Check sheet for the modelled part. Datum: model origin and axes. Units: mm. A direction names the side the tool comes from. Give positions to 0.01 mm unless a question says otherwise; leave off trailing zeros. Order: outer loops, then holes, each group sorted by start corner. A loop starts at its lowest first (then second) coordinate and runs counter-clockwise, first axis right, second up. Notation, with made-up numbers: (31, -9.75) -> (77, -9.75) arc R17 cw to (77, -5.75) -> close; hole circle Ø11 at (16, 29.25). An arc over 180 degrees is marked (long way). One line per question, with ' | ' between items.
```python
from build123d import *

# Parameters (mm, degrees)
AUFSATZ_LINEAR_AUSTRAGEN3_DEPTH      = 20
SKIZZE10_OUTSIDE_W                   = 46.486
SKIZZE10_OUTSIDE_H                   = 31.486
SCHNITT_LINEAR_AUSTRAGEN9_DEPTH      = 13.5
SCHNITT_LINEAR_AUSTRAGEN9_DEPTH_BACK = 13.5
SKIZZE7_R                            = 1.23
SCHNITT_LINEAR_AUSTRAGEN8_DEPTH      = 12


with BuildPart() as part:
    # Skizze3 → Aufsatz-Linear austragen3 (new body)
    with BuildSketch(Plane.XY):
        with BuildLine():
            Line((-17.5, 4), (-2.308809744, 11.933429348))
            ThreePointArc((-2.308809744, 11.933429348), (0, 12.5), (2.308809744, 11.933429348))
            Line((2.308809744, 11.933429348), (17.5, 4))
            Line((17.5, 4), (17.5, -4))
            Line((17.5, -4), (2.308809744, -11.933429348))
            ThreePointArc((2.308809744, -11.933429348), (0, -12.5), (-2.308809744, -11.933429348))
            Line((-2.308809744, -11.933429348), (-17.5, -4))
            Line((-17.5, -4), (-17.5, 4))
        make_face()
        with BuildLine():
            Line((-2.25, -7.51244486), (-2.25, 7.51244486))
            ThreePointArc((-2.25, 7.51244486), (0, 9.76244486), (2.25, 7.51244486))
            Line((2.25, 7.51244486), (2.25, -7.51244486))
            ThreePointArc((2.25, -7.51244486), (0, -9.76244486), (-2.25, -7.51244486))
        make_face(mode=Mode.SUBTRACT)
    extrude(amount=AUFSATZ_LINEAR_AUSTRAGEN3_DEPTH)

    # Skizze10 outside → Schnitt-Linear austragen9 (cut, two sides)
    with BuildSketch(Plane(origin=(0, 0, 0), x_dir=(1, 0, 0), z_dir=(0, 1, 0))) as schnitt_linear_austragen9_sk:
        with Locations((0, -10)):
            Rectangle(SKIZZE10_OUTSIDE_W, SKIZZE10_OUTSIDE_H)
        with BuildLine():
            Line((-16.110814579, 0), (-17.5, -7.878462024))
            Line((-17.5, -7.878462024), (-3.472963553, -10.351807009))
            ThreePointArc((-3.472963553, -10.351807009), (0, -10.655651949), (3.472963553, -10.351807009))
            Line((3.472963553, -10.351807009), (17.5, -7.878462024))
            Line((17.5, -7.878462024), (16.110814579, 0))
            Line((16.110814579, 0), (-16.110814579, 0))
        make_face(mode=Mode.SUBTRACT)
    extrude(amount=SCHNITT_LINEAR_AUSTRAGEN9_DEPTH, mode=Mode.SUBTRACT)
    extrude(schnitt_linear_austragen9_sk.sketch, amount=-SCHNITT_LINEAR_AUSTRAGEN9_DEPTH_BACK, mode=Mode.SUBTRACT)

    # Skizze7 → Schnitt-Linear austragen8 (cut)
    with BuildSketch(Plane(origin=(-16.983254832, 0, 4.947854546), x_dir=(-0.173648178, 0, 0.984807753), z_dir=(-0.984807753, 0, -0.173648178))):
        with Locations((-1.524183177, 0)):
            Circle(SKIZZE7_R)
    schnitt_linear_austragen8 = extrude(amount=-SCHNITT_LINEAR_AUSTRAGEN8_DEPTH, mode=Mode.SUBTRACT)

    # Spiegeln4: Schnitt-Linear austragen8 across plane
    add(schnitt_linear_austragen8.mirror(Plane(origin=(0, 0, 0), x_dir=(0, 0, 1), z_dir=(1, 0, 0))), mode=Mode.SUBTRACT)


solid = part.part
```
Q1. Section check B-B (y = 2.5). Enter the section's corners in (x, z), and give its area (3 significant figures).
Result sheet:
outline: (-17.5, 7.88) -> (-16.11, 0) -> (-2.25, 0) -> (-2.25, 10.53) arc R20 ccw to (-3.47, 10.35) -> close; (2.25, 0) -> (16.11, 0) -> (17.5, 7.88) -> (3.47, 10.35) arc R20 ccw to (2.25, 10.53) -> close | area: 270 mm2
Q2. Depth check by flat-ended pin: pin 1 Ø1 at (y, z) = (8, 5.5) entering from +X; pin 2 Ø6 at (x, z) = (1, 5) entering from +Y; pin 3 Ø5 at (x, z) = (6.5, 5.5) entering from +Y; pin 4 Ø3 at (y, z) = (1, 4) entering from +X. Enter the tip coordinate at first touch or a pass-through.
Result sheet:
pin 1: stops at x = 10.8 | pin 2: stops at y = 12.5 | pin 3: stops at y = 11.05 | pin 4: stops at x = 17.08
Q3. Section check A-A (x = 0). Enter the section's corners in (y, z), and give its area (3 significant figures).
Result sheet:
outline: (-12.5, 0) -> (-9.76, 0) -> (-9.76, 10.66) -> (-12.5, 10.66) -> close; (9.76, 0) -> (12.5, 0) -> (12.5, 10.66) -> (9.76, 10.66) -> close | area: 58.3 mm2
Q4. Section check C-C (z = 9.75). Enter the section's corners in (x, y), and give its area (3 significant figures).
Result sheet:
outline: (-6.89, -9.54) -> (-2.31, -11.93) arc R4.99 ccw to (2.31, -11.93) -> (6.89, -9.54) -> (6.89, 9.54) -> (2.31, 11.93) arc R4.99 ccw to (-2.31, 11.93) -> (-6.89, 9.54) -> close; hole (-2.25, -7.51) arc R2.25 ccw to (2.25, -7.51) -> (2.25, 7.51) arc R2.25 ccw to (-2.25, 7.51) -> close | area: 227 mm2
Q5. Access from +Z, -Z, +X, -X, +Y, -Y to the whole of each face (thin tool, end or side, straight path). Record for faces 5 (the face through (0, -12.5, 5.3)), 6 (the face through (-0.05, 9.76, 5.25)).
Result sheet:
face 5: +Z, -Z, -Y | face 6: +Z, -Z
Q6. Section check D-D (y = -0.5). Enter the section's corners in (x, z), and give its area (3 significant figures).
Result sheet:
outline: (-17.5, 7.88) -> (-16.91, 4.55) -> (-5.1, 6.64) -> (-4.71, 4.42) -> (-16.52, 2.34) -> (-16.11, 0) -> (-2.25, 0) -> (-2.25, 10.53) arc R20 ccw to (-3.47, 10.35) -> close; (2.25, 0) -> (16.11, 0) -> (16.52, 2.34) -> (4.71, 4.42) -> (5.1, 6.64) -> (16.91, 4.55) -> (17.5, 7.88) -> (3.47, 10.35) arc R20 ccw to (2.25, 10.53) -> close | area: 216 mm2
Q7. Mould release check, pull along Z, two halves, no side actions. Record for faces 1 (the face through (-10.01, 7.91, 5.19)), 2 (the face through (4.898, 0.017, 5.514)), 3 (the face through (-16.95, 0.98, 4.76)), 4 (the face through (-11.1, 0.37, 5.63)): pulls with the +Z half, pulls with the -Z half, needs draft (parallel to the pull), parting line crosses it, or undercut.
Result sheet:
face 1: needs draft | face 2: undercut | face 3: pulls with the -Z half | face 4: undercut
Q8. Thickness scan on line 1 (Y direction, x = 0, z = 6.5); line 2 (X direction, y = -2, z = 1.75); line 3 (Y direction, x = -10.5, z = 5.25). Record the ranges inside material, lowest first.
Result sheet:
line 1: y = -12.5 to -9.76, 9.76 to 12.5 | line 2: x = -16.42 to -2.25, 2.25 to 16.42 | line 3: y = -7.66 to -1.01, 1.01 to 7.66
